Here's how the part is built. I have some questions about the finished solid (model axes, mm). A direction names the side the tool comes from. Round coordinates to 2 decimals unless told otherwise and drop trailing zeros. Loops run counter-clockwise (first coordinate to the right, second up) from the corner with the lowest first, then second, coordinate; pieces in that order, holes last. Notation, with made-up numbers: M -6,8.25 L 19,8.25 A28 cw 19,41.25 Z; hole C -2,-35 d3. An arc over 180 degrees is marked long. Use a Markdown table: item, result.
from build123d import *

# Parameters (mm, degrees)
F1_DEPTH = 400
F3_DEPTH = 290.001
F5_DEPTH = 161.870333055


# Not quite as in the source:
# - a feature names something its author has since deleted; it is built from what else it names


with BuildPart() as f1:
    # F0 (on Right) → F1 (new body)
    with BuildSketch(Plane.YZ):
        Polygon((-80, 0), (0, 0), (0, 501), (-1, 501), (-1, 1), (-79.5336923418, 1), (-289, 250.6322246791), (-289, 501), (-290, 501), (-290, 250.2682544448), align=None)
    extrude(amount=-F1_DEPTH)

    # F2 (on face) → F3 (cut, through all)
    with BuildSketch(Plane(origin=(0, 0, 0), x_dir=(-1, 0, 0), z_dir=(0, 1, 0))):
        Polygon((400, 0), (400, 240), (250, 80), (250, 0), align=None)
        Polygon((0, 0), (150, 0), (150, 80), (0, 240), align=None)
    extrude(amount=-F3_DEPTH, mode=Mode.SUBTRACT)

    # F4 (on face) → F5 (cut, through all)
    with BuildSketch(Plane(origin=(0, -46.1798826636, -38.7495225108), x_dir=(-1, 0, 0), z_dir=(0, 0.7660444431, 0.6427876097))):
        with BuildLine():
            Line((180, 116.8893164331), (180, 76.8893164331))
            ThreePointArc((180, 76.8893164331), (200, 56.8893164331), (220, 76.8893164331))
            Line((220, 76.8893164331), (220, 116.8893164331))
            ThreePointArc((220, 116.8893164331), (200, 136.8893164331), (180, 116.8893164331))
        make_face()
    extrude(amount=-F5_DEPTH, mode=Mode.SUBTRACT)


solid = f1.part
1. For pin 1 Ø12 at (x, y) = (-172, -116.5) entering from +Z; pin 2 Ø8 at (y, z) = (-108.5, 32.5) entering from +X; pin 3 Ø8 at (y, z) = (-197, 144.5) entering from -X, each with a flat end and sliding along its axis, tell me the tip position at first contact or that it passes through.
Answer sheet:
| item | result |
|---|---|
| pin 1 | z = 52.21 |
| pin 2 | x = -150 |
| pin 3 | x = -311.48 |
2. I need wall thicknesses on probe 1 along Y at (x, z) = (-141, 363); probe 2 along Y at (x, z) = (-230.5, 236); probe 3 along Z at (x, y) = (-160, -108). Which ranges of each line are inside material? Lowest first, please. Write a range as from..to.
Answer sheet:
| item | result |
|---|---|
| probe 1 | -290..-289, -1..0 |
| probe 2 | -278.03..-276.72, -1..0 |
| probe 3 | 33.37..34.92 |
3. Imagine slicing it at D-D, the plane y = -51. Write out the boundary of the cut face in (x, z), then the cut area to 3 significant figures.
Answer sheet:
| item | result |
|---|---|
| outline | M -250,0 L -150,0 L -150,1 L -250,1 Z |
| area | 100 mm2 |
4. Imagine slicing it at A-A, the plane z = 300. Write out the boundary of the cut face in (x, y).
Answer sheet:
| item | result |
|---|---|
| outline | M -400,-290 L 0,-290 L 0,-289 L -400,-289 Z; M -400,-1 L 0,-1 L 0,0 L -400,0 Z |
5. We'd pull the mould along Y, two halves only. Please class faces 4 (the face through (-75.35, -213.287, 159.627)), 5 (the face through (-197.2, -206.075, 151.806)), 6 (the face through (-200.44, -134.55, 65.79)), 7 (the face through (-197, -290, 377)): +Y half, -Y half, draft (parallel to the pull), parting line (faces both ways), or undercut.
Answer sheet:
| item | result |
|---|---|
| face 4 | draft |
| face 5 | undercut |
| face 6 | undercut |
| face 7 | -Y half |
6. Imagine slicing it at C-C, the plane z = 35. Write out the boundary of the cut face in (x, y).
Answer sheet:
| item | result |
|---|---|
| outline | M -250,-109.37 L -220,-109.37 L -220,-108.06 L -250,-108.06 Z; M -250,-1 L -150,-1 L -150,0 L -250,0 Z; M -180,-109.37 L -150,-109.37 L -150,-108.06 L -180,-108.06 Z |
7. Imagine slicing it at B-B, the plane x = -126. Write out the boundary of the cut face in (y, z), then the cut area to 3 significant figures.
Answer sheet:
| item | result |
|---|---|
| outline | M -290,250.27 L -168.61,105.6 L -167.3,105.6 L -289,250.63 L -289,501 L -290,501 Z; M -1,105.6 L 0,105.6 L 0,501 L -1,501 Z |
| area | 835 mm2 |
8. Which directions (+Z, -Z, +X, -X, +Y, -Y) give clear straight access to the entire face, cutting with the end or side of a thin tool? Please do faces 1 (the face through (-180, -109, 35)), 2 (the face through (-76.05, -0.49, 158.88)), 3 (the face through (-199, -40, 1)).
Answer sheet:
| item | result |
|---|---|
| face 1 | +Z, -Z, -Y |
| face 2 | -Z, +X, +Y, -Y |
| face 3 | +Z, +X, -X |
